Geometry: final body of the model. Coordinates: model frame, mm. A direction names the side the tool comes from. Round coordinates to 2 decimals unless told otherwise and drop trailing zeros. Write each loop counter-clockwise with the first axis right and the second up, starting at its lowest first coordinate (ties: lowest second). Pieces come first, ordered by that corner, then holes. Notation, with made-up numbers: M 17,1 L 42,1 A26 ccw 42,19 Z; hole C 80.25,3 d4. An arc over 180 degrees is marked long. Use one line per item in the form item = value. Start each with the question number.
Item 1: Ray query, probe 1 along Z at (x, y) = (0.1, -4.6); probe 2 along Y at (x, z) = (-5, 10); probe 3 along Z at (x, y) = (0.5, -7.25). Return the intervals inside material, ascending.
Item 2: Section query B-B (x = 0.1). State how many separate pieces and enclosed holes the cut face has, and give its area (3 significant figures).
Item 3: Pin query (flat end, axial travel): pin 1 Ø2 at (x, z) = (-1, 13.5) entering from +Y; pin 2 Ø2 at (x, z) = (0, 4) entering from +Y. Return the tip coordinate at first contact, or that it passes through.
Item 4: Pull-direction query (Z, two-part tool) for faces 1 (the flat face through (0, -4, 50)), 2 (the flat face through (-2, -3.5, 45)), 3 (the flat face through (3, -7.8, 25)); classes: pulls with the +Z half, pulls with the -Z half, needs draft (parallel to the pull), parting line crosses it, or undercut.
Item 5: Section query D-D (x = 3). Return loops of the section in (y, z).
Item 6: Reachability of faces 4 (the flat face through (0, -4, 0)), 5 (the flat face through (-2, -3.5, 5)) from +Z, -Z, +X, -X, +Y, -Y: full face, straight path, thin tool, end or side. Return the list, or none.
Item 7: Section query C-C (x = -2.25). Return loops of the section in (y, z).
Autodesk Inventor part; units mm, degrees
ref_plane "YZ Plane" through (0, 0, 0) normal (1, 0, 0) x (0, 1, 0)
ref_plane "XZ Plane" through (0, 0, 0) normal (0, 1, 0) x (-1, 0, 0)
ref_plane "XY Plane" through (0, 0, 0) normal (0, 0, 1) x (1, 0, 0)
ref_plane "Work Plane1" through (0, 0, 0) normal (0, 0, 1) x (1, 0, 0)
sketch "Sketch1" plane through (0, 0, 0) normal (0, 0, 1) x (1, 0, 0)
  line L0 (0, 0) -> (5.55, 0)
  line L1 (6.05, -7.8) -> (0, -7.8)
  line L2 (0, -7.8) -> (0, 0)
  line L3 (5.55, 0) -> (6.05, -0.5)
  arc A0 (6.05, -3.6294) -> (5.8482, -3.4873) centre (5.8013, -3.7683) ccw
  arc A1 (5.5514, -3.0941) -> (5.8482, -3.4873) centre (6.6343, -2.5853) ccw
  arc A2 (5.5514, -3.0941) -> (5.425, -2.9829) centre (5.3332, -3.2146) ccw
  line L4 (5.425, -2.9829) -> (4.928, -2.9441)
  arc A3 (4.7, -2.7255) -> (4.928, -2.9441) centre (4.9475, -2.6956) ccw
  arc A4 (4.9275, -2.0261) -> (4.7, -2.2744) centre (4.9493, -2.2744) ccw
  arc A5 (5.293, -1.9942) -> (5.5514, -1.8412) centre (5.3208, -1.7464) ccw
  arc A6 (5.8954, -1.3233) -> (5.5514, -1.8412) centre (6.7024, -2.2326) ccw
  arc A7 (5.8954, -1.3233) -> (6.05, -1.1) centre (5.8008, -1.0927) ccw
  line L5 (5.293, -1.9942) -> (4.9275, -2.0261)
  line L6 (4.7, -2.7255) -> (4.7, -2.2744)
  line L7 (6.05, -0.5) -> (6.05, -1.1)
  line L8 (6.05, -3.6294) -> (6.05, -7.8)
  point P0 (6.05, 0)
  dimension "d0" = 0.5
  dimension "d1" = 0.5
  dimension "d17" = 6.05
  dimension "d18" = 7.8
  dimension "d20" = 2.6756
  dimension "d21" = 0.5
  dimension "d22" = 1.1
  dimension "d23" = 4.7
  dimension "d24" = 0.2275
  dimension "d25" = 0.228
  dimension "d26" = 0
  dimension "d27" = 0.2483
  dimension "d28" = 0.2186
extrude "Extrusion1" add sketch "Sketch1" along normal blind 50
mirror "Mirror1" about plane through (0, 0, 0) normal (-1, 0, 0) of "Extrusion1"
sketch "Sketch2" plane through (5.55, 0, 50) normal (0, 1, 0) x (1, 0, 0)
  line L0 (-11.1, 50) -> (0, 50)
  line L1 (-11.1, 50) -> (-11.1, 0)
  line L2 (0, 0) -> (-11.1, 0)
  line L3 (0, 50) -> (0, 0)
  point P0 (-5.55, 50)
  point P1 (-5.45, 45.5983)
hole "Hole1" at (0.1, 0, 4.4017) direction (0, -1, 0) diameter 3.5 end through all counterbore diameter 7 counterbore depth 3.5
pattern_linear "Rectangular Pattern1" count 5 spacing 10 along (0, 0, 1) of "Hole1"
ref_plane "Work Plane2" through (0, -7.8, 0) normal (1, 0, 0) x (0, 0, -1)
properties part number "30_Cube_Z_Focus_MGN_NEMA_rail"
Working result:
q1.probe_1 = 0 to 2.65, 6.15 to 12.65, 16.15 to 22.65, 26.15 to 32.65, 36.15 to 42.65, 46.15 to 50
q1.probe_2 = -7.8 to -2.95, -2.02 to 0
q1.probe_3 = 0 to 2.7, 6.11 to 12.7, 16.11 to 22.7, 26.11 to 32.7, 36.11 to 42.7, 46.11 to 50
q2.separate_pieces = 6
q2.enclosed_holes = 0
q2.area = 192 mm²
q3.pin_1 = -3.5
q3.pin_2 = through
q4.face_1 = pulls with the +Z half
q4.face_2 = undercut
q4.face_3 = needs draft
q5.outline = M -7.8,0 L 0,0 L 0,2.44 L -3.5,2.44 L -3.5,6.36 L 0,6.36 L 0,12.44 L -3.5,12.44 L -3.5,16.36 L 0,16.36 L 0,22.44 L -3.5,22.44 L -3.5,26.36 L 0,26.36 L 0,32.44 L -3.5,32.44 L -3.5,36.36 L 0,36.36 L 0,42.44 L -3.5,42.44 L -3.5,46.36 L 0,46.36 L 0,50 L -7.8,50 Z
q6.face_4 = -Z, +X, -X, +Y, -Y
q6.face_5 = +Y
q7.outline = M -7.8,0 L 0,0 L 0,1.81 L -3.5,1.81 L -3.5,7 L 0,7 L 0,11.81 L -3.5,11.81 L -3.5,17 L 0,17 L 0,21.81 L -3.5,21.81 L -3.5,27 L 0,27 L 0,31.81 L -3.5,31.81 L -3.5,37 L 0,37 L 0,41.81 L -3.5,41.81 L -3.5,47 L 0,47 L 0,50 L -7.8,50 Z
